Part print with two shaded views. Sizes in mm from the minimum x, y, z corner. A direction names the side the tool comes from. Round coordinates to 2 decimals unless told otherwise and drop trailing zeros. Order: outer loops, then holes, each group sorted by start corner. A loop starts at its lowest first (then second) coordinate and runs counter-clockwise, first axis right, second up. Notation, with made-up numbers: (32, 28.25) -> (63, 28.25) arc R21 cw to (63, 66.25) -> close; hole circle Ø2 at (-32, 28.25). An arc over 180 degrees is marked (long way). Answer as a JSON object with one key per item and string values.
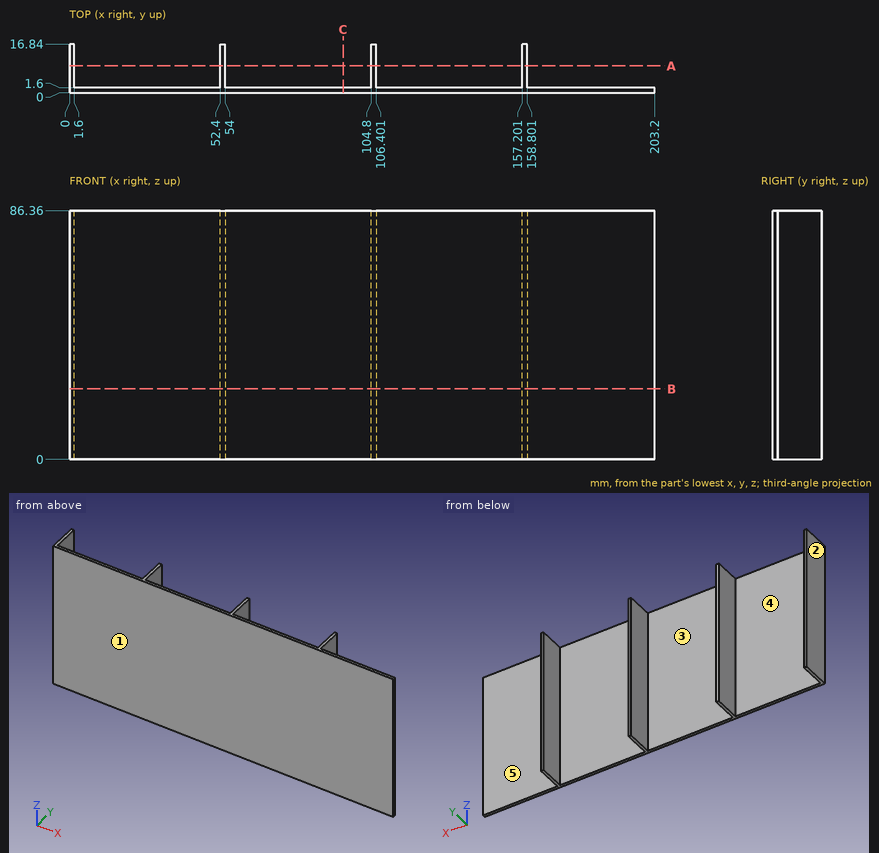
1) Cut at A-A, the plane y = 9.25. Give the cut face in (x, z).
Checked values:
{"outline": "(0, 0) -> (1.6, 0) -> (1.6, 86.36) -> (0, 86.36) -> close; (52.4, 0) -> (54, 0) -> (54, 86.36) -> (52.4, 86.36) -> close; (104.8, 0) -> (106.4, 0) -> (106.4, 86.36) -> (104.8, 86.36) -> close; (157.2, 0) -> (158.8, 0) -> (158.8, 86.36) -> (157.2, 86.36) -> close"}
2) Flat gauge pins, fed straight in: pin 1 Ø15 at (x, z) = (87, 52.5) entering from +Y; pin 2 Ø5 at (y, z) = (11.5, 17.5) entering from +X. Where does each tip first touch, or does it go through?
Checked values:
{"pin 1": "stops at y = 1.6", "pin 2": "stops at x = 158.8"}
3) Which spindle directions (+Z, -Z, +X, -X, +Y, -Y) get a long thin tool onto all of the face, cutting with end or side? Do the marked faces 4 and 5. Say none if no direction does.
Checked values:
{"face 4": "+Z, -Z, +Y", "face 5": "+Z, -Z, +X, +Y"}
4) Pull direction X, two halves, no side cores. Call the marked faces 1, 2 and 3: pulls with the +X half, pulls with the -X half, needs draft (parallel to the pull), parting line crosses it, or undercut.
Checked values:
{"face 1": "needs draft", "face 2": "pulls with the -X half", "face 3": "undercut"}
5) Probe L1, parallel to X at y = 14.75, z = 73; L2, parallel to Y at x = 85, z = 67.5. List the from-to ranges inside material, lowest first. Write a range as from..to.
Checked values:
{"L1": "x = 0..1.6, 52.4..54, 104.8..106.4, 157.2..158.8", "L2": "y = 0..1.6"}
6) Cut at C-C, the plane x = 95. Give the cut face in (y, z).
Checked values:
{"outline": "(0, 0) -> (1.6, 0) -> (1.6, 86.36) -> (0, 86.36) -> close"}
7) Cut at B-B, the plane z = 24.5. Give the cut face in (x, y).
Checked values:
{"outline": "(0, 0) -> (203.2, 0) -> (203.2, 1.6) -> (158.8, 1.6) -> (158.8, 16.84) -> (157.2, 16.84) -> (157.2, 1.6) -> (106.4, 1.6) -> (106.4, 16.84) -> (104.8, 16.84) -> (104.8, 1.6) -> (54, 1.6) -> (54, 16.84) -> (52.4, 16.84) -> (52.4, 1.6) -> (1.6, 1.6) -> (1.6, 16.84) -> (0, 16.84) -> close"}
